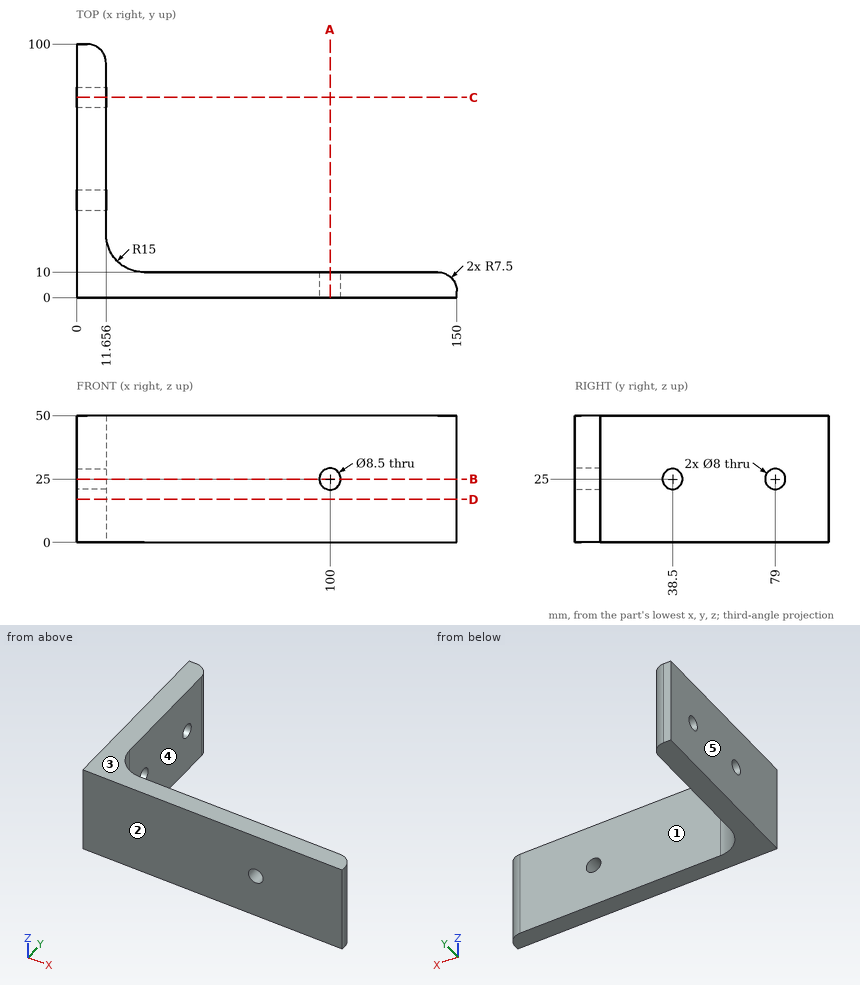
Source: three-view drawing plus pictorial views. Frame: mm from the lowest corner of the part. A direction names the side the tool comes from. Coordinates: 2 decimals unless noted, no trailing zeros. Loops run counter-clockwise (first coordinate to the right, second up) from the corner with the lowest first, then second, coordinate; pieces in that order, holes last. Notation, with made-up numbers: (59.5, 42.25) - (77.5, 42.25) arc R29 cw to (77.5, 76.25) - close; hole circle Ø1 at (77, -26). An arc over 180 degrees is marked (long way). One line per item, written item: value. Start each with the question number.
1. Section B-B (z = 25). Return the cut outline in (x, y), and give its area (3 significant figures).
2. Contact query for a flat-ended pin moving along its axis: P1, Ø10, axis at y = 66, z = 21, coming from the +X side. Output: stop coordinate, or through.
3. Mould query, pull axis Y, two halves, no side actions, for the marked faces 1, 2 and 3. Classes: pulls with the +Y half, pulls with the -Y half, needs draft (parallel to the pull), parting line crosses it, or undercut.
4. Section D-D (z = 17). Return the cut outline in (x, y), and give its area (3 significant figures).
5. Section A-A (x = 100). Return the cut outline in (y, z).
6. Set-up query: the marked faces 4 and 5. Return all of +Z, -Z, +X, -X, +Y, -Y with unobstructed straight access to the full face (end or side cutting, diameter ignored); none if empty.
7. Section C-C (y = 79). Return the cut outline in (x, z).
8. Ray query, L1, parallel to Y at x = 10.5, z = 24.5; L2, parallel to Z at x = 6, y = 38; L3, parallel to Y at x = 8.5, z = 25 (1 decimal). Return the intervals inside material, ascending.
Verdict:
1. outline: (0, 0) - (95.75, 0) - (95.75, 10) - (26.66, 10) arc R15 cw to (11.66, 25) - (11.66, 34.5) - (0, 34.5) - close; (0, 42.5) - (11.66, 42.5) - (11.66, 75) - (0, 75) - close; (0, 83) - (11.66, 83) - (11.66, 92.5) arc R7.5 ccw to (4.16, 100) - (0, 100) - close; (104.25, 0) - (150, 0) - (150, 2.5) arc R7.5 ccw to (142.5, 10) - (104.25, 10) - close
1. area: 2,300 mm2
2. P1: stops at x = 11.66
3. face 1: pulls with the +Y half
3. face 2: pulls with the -Y half
3. face 3: needs draft
4. outline: (0, 0) - (150, 0) - (150, 2.5) arc R7.5 ccw to (142.5, 10) - (26.66, 10) arc R15 cw to (11.66, 25) - (11.66, 92.5) arc R7.5 ccw to (4.16, 100) - (0, 100) - close
4. area: 2,570 mm2
5. outline: (0, 0) - (10, 0) - (10, 20.75) - (0, 20.75) - close; (0, 29.25) - (10, 29.25) - (10, 50) - (0, 50) - close
6. face 4: +Z, -Z, +X, +Y
6. face 5: +Z, -Z, -X, +Y, -Y
7. outline: (0, 0) - (11.66, 0) - (11.66, 21) - (0, 21) - close; (0, 29) - (11.66, 29) - (11.66, 50) - (0, 50) - close
8. L1: y = 0 to 34.53, 42.47 to 75.03, 82.97 to 96.5
8. L2: z = 0 to 21.03, 28.97 to 50
8. L3: y = 0 to 34.5, 42.5 to 75, 83 to 98.6
